Could you check a few things on this model? Use its own coordinates, in mm. Give positions to 0.01 mm unless a question says otherwise; leave off trailing zeros. Order: outer loops, then holes, each group sorted by start corner. A loop starts at its lowest first (then second) coordinate and runs counter-clockwise, first axis right, second up.
from build123d import *

# Parameters (mm, degrees)
BOSS_EXTRUDE1_DEPTH = 5
TAPPED_HOLE1_D      = 5


with BuildPart() as part:
    # Sketch1 → Boss-Extrude1 (new body)
    with BuildSketch(Plane(origin=(0, 0, 0), x_dir=(1, 0, 0), z_dir=(0, 1, 0))):
        Polygon((0, 5.773502692), (-5, 2.886751346), (-5, -2.886751346), (0, -5.773502692), (5, -2.886751346), (5, 2.886751346), align=None)
    extrude(amount=-BOSS_EXTRUDE1_DEPTH)

    # Sketch2 → Cut-Revolve1 (revolve, cut)
    with BuildSketch(Plane(origin=(0, 0, 0), x_dir=(0, 0, -1), z_dir=(1, 0, 0))):
        Polygon((5, 0), (5.773502692, 0), (5.773502692, -0.446581987), align=None)
    revolve(axis=Axis((0, 0, 0), (0, -1, 0)), mode=Mode.SUBTRACT)

    # Tapped Hole1 (through all)
    with Locations(Plane(origin=(0, 0, 0), x_dir=(1, 0, 0), z_dir=(0, 1, 0))):
        with Locations((0, 0)):
            Hole(TAPPED_HOLE1_D / 2)


solid = part.part
Item 1: We'd pull the mould along Z, two halves only. Please class faces 1 (the flat face through (2.465, -2.465, 4.35)), 2 (the cylindrical face through (0.54, -2.54, 2.44)), 3 (the flat face through (2, 0, 2)), 4 (the flat face through (2.535, -2.465, -4.31)): +Z half, -Z half, draft (parallel to the pull), parting line (faces both ways), or undercut.
Findings:
face 1: +Z half
face 2: undercut
face 3: draft
face 4: -Z half
Item 2: Imagine slicing it at A-A on y = -4.55. List the corners of the cut face in (x, z) for me, then the cut area to 3 significant figures.
Findings:
outline: (-5, -2.89) - (0, -5.77) - (5, -2.89) - (5, 2.89) - (0, 5.77) - (-5, 2.89) - close; hole circle Ø5 at (0, 0)
area: 67.0 mm2
Item 3: Please list where these lines run through material, in increasing order: line 1 along Z through (x, y) = (1, -1.75); line 2 along Z through (x, y) = (-0.5, -4.55); line 3 along X through (y, z) = (-2.05, 0.5).
Findings:
line 1: z = -5.2 to -2.29, 2.29 to 5.2
line 2: z = -5.48 to -2.45, 2.45 to 5.48
line 3: x = -5 to -2.45, 2.45 to 5
Item 4: For pin 1 (1.5 mm diameter, centred on x = -0.5, y = -2, fed in from +Z); pin 2 (3 mm diameter, centred on x = -2.5, y = -4.5, fed in from -Z); pin 3 (3 mm diameter, centred on x = 0, z = 0, fed in from +Y), each with a flat end and sliding along its axis, tell me the tip position at first contact or that it passes through.
Findings:
pin 1: stops at z = 5.77
pin 2: stops at z = -5.2
pin 3: passes through
